from build123d import *

# Parameters (mm, degrees)
F1_DEPTH = 10
F2_SIZE  = 0.2


with BuildPart() as f1:
    # F0 (on Front) → F1 (new body)
    with BuildSketch(Plane.XZ):
        Polygon((-45.385001, 10), (-55.385001, 10), (-55.385001, 0), (58.614999, 0), (58.614999, 10), (48.614999, 10), (48.614999, 5), (38.614999, 5), (38.614999, 10), (-35.385001, 10), (-35.385001, 5), (-45.385001, 5), align=None)
    extrude(amount=F1_DEPTH)

    # F2
    f2_edges = [f1.edges().sort_by_distance(p)[0] for p in [
        (-40.385001, -10, 5),
        (-45.385001, -10, 7.5),
        (-50.385001, -10, 10),
        (-55.385001, -10, 5),
        (1.614999, -10, 0),
        (58.614999, -10, 5),
        (53.614999, -10, 10),
        (48.614999, -10, 7.5),
        (43.614999, -10, 5),
        (38.614999, -10, 7.5),
        (1.614999, -10, 10),
        (-35.385001, -10, 7.5),
        (38.614999, -5, 10),
        (-35.385001, -5, 10),
        (1.614999, 0, 10),
        (-35.385001, -5, 5),
        (-45.385001, -5, 5),
        (-40.385001, 0, 5),
        (-45.385001, -5, 10),
        (-55.385001, -5, 10),
        (-50.385001, 0, 10),
        (-45.385001, 0, 7.5),
        (-55.385001, 0, 5),
        (1.614999, 0, 0),
        (58.614999, 0, 5),
        (53.614999, 0, 10),
        (48.614999, 0, 7.5),
        (43.614999, 0, 5),
        (38.614999, 0, 7.5),
        (-35.385001, 0, 7.5),
        (58.614999, -5, 0),
        (58.614999, -5, 10),
        (48.614999, -5, 10),
        (48.614999, -5, 5),
        (-55.385001, -5, 0),
    ]]
    chamfer(f2_edges, length=F2_SIZE)


solid = f1.part
The listing builds one solid part. Answer for the finished solid, in the listing's coordinates (mm). A direction names the side the tool comes from. Round coordinates to 2 decimals unless told otherwise and drop trailing zeros. Write each loop counter-clockwise with the first axis right and the second up, starting at its lowest first coordinate (ties: lowest second). Pieces come first, ordered by that corner, then holes. Notation, with made-up numbers: M 80.25,76 L 101.25,76 A29 ccw 101.25,115 Z; hole C 11.5,21 d11. An arc over 180 degrees is marked long. Write each question's results on one line, items separated by ' | '. Start each with the question number.
(1) Find the intervals of material crossed by line 1 (X direction, y = -5, z = 8.25) (3 decimals); line 2 (Z direction, x = -42, y = -2.5), in increasing order.
(2) The part is cut by section A-A, the plane z = 7.25. Write down the section's boundary in (x, y) (3 decimals).
(3) Determine the mould class of faces 1 (the flat face through (58.615, -5, 5)), 2 (the flat face through (48.615, -5, 8)), 3 (the flat face through (1, -5, 0)) for opening direction X: +X half, -X half, draft (parallel to the pull), parting line (faces both ways), or undercut.
(4) This flat-tipped pin is pushed along its axis until it touches: P1, Ø3, axis at x = -39, y = -3, coming from the +Z side. Where does it stop, or does it pass through?
(5) For faces 4 (the flat face through (-55.385, -5, 5)), 5 (the flat face through (-45.385, -5, 7)), determine the directions among +Z, -Z, +X, -X, +Y, -Y from which every point of the face is accessible in a straight line to the end or side of a thin tool.
(6) The part is cut by section B-B, the plane y = -5.25. Write down the section's boundary in (x, z) (3 decimals).
Worked answers:
1) line 1: x = -55.385 to -45.385, -35.385 to 38.615, 48.615 to 58.615 | line 2: z = 0 to 5
2) outline: M -55.385,-9.8 L -55.185,-10 L -45.585,-10 L -45.385,-9.8 L -45.385,-0.2 L -45.585,0 L -55.185,0 L -55.385,-0.2 Z; M -35.385,-9.8 L -35.185,-10 L 38.415,-10 L 38.615,-9.8 L 38.615,-0.2 L 38.415,0 L -35.185,0 L -35.385,-0.2 Z; M 48.615,-9.8 L 48.815,-10 L 58.415,-10 L 58.615,-9.8 L 58.615,-0.2 L 58.415,0 L 48.815,0 L 48.615,-0.2 Z
3) face 1: +X half | face 2: undercut | face 3: draft
4) P1: stops at z = 5
5) face 4: +Z, -Z, -X, +Y, -Y | face 5: +Z, +Y, -Y
6) outline: M -55.385,0.2 L -55.185,0 L 58.415,0 L 58.615,0.2 L 58.615,9.8 L 58.415,10 L 48.815,10 L 48.615,9.8 L 48.615,5.2 L 48.415,5 L 38.615,5 L 38.615,9.8 L 38.415,10 L -35.185,10 L -35.385,9.8 L -35.385,5.2 L -35.585,5 L -45.185,5 L -45.385,5.2 L -45.385,9.8 L -45.585,10 L -55.185,10 L -55.385,9.8 Z
